Read the model definition and answer for the solid it produces. Units are mm, in the model's axes. A direction names the side the tool comes from. Give positions to 0.01 mm unless a question says otherwise; leave off trailing zeros. Order: outer loops, then holes, each group sorted by start corner. A loop starts at its lowest first (then second) coordinate and runs counter-clockwise, first axis right, second up. Notation, with made-up numbers: (18.5, -13.5) - (36.5, -13.5) arc R23 ccw to (36.5, 2.5) - close; hole circle Ø3 at (-22.75, 13). An arc over 180 degrees is marked (long way). Return JSON: item names as keys, results as strings.
```python
from build123d import *

# Parameters (mm, degrees)
SKETCH1_R           = 1.6
BOSS_EXTRUDE1_DEPTH = 1.65
SKETCH2_W           = 16.5
SKETCH2_H           = 12.1
BOSS_EXTRUDE2_DEPTH = 11


with BuildPart() as part:
    # Sketch1 → Boss-Extrude1 (new body)
    with BuildSketch(Plane(origin=(0, 0, 0), x_dir=(1, 0, 0), z_dir=(0, 1, 0))):
        Polygon((99.1, 0), (99.1, 1), (101.6, 3.5), (101.6, 43.3), (99.1, 45.8), (99.1, 50.8), (96.6, 53.3), (0, 53.3), (0, 0), align=None)
        with Locations((15.524, 50.76)):
            Circle(SKETCH1_R, mode=Mode.SUBTRACT)
        with Locations((14, 2.5)):
            Circle(SKETCH1_R, mode=Mode.SUBTRACT)
        with Locations((96.55, 2.5)):
            Circle(SKETCH1_R, mode=Mode.SUBTRACT)
        with Locations((90.454, 50.76)):
            Circle(SKETCH1_R, mode=Mode.SUBTRACT)
        with Locations((66.1, 35.5)):
            Circle(SKETCH1_R, mode=Mode.SUBTRACT)
        with Locations((66.1, 7.6)):
            Circle(SKETCH1_R, mode=Mode.SUBTRACT)
    extrude(amount=BOSS_EXTRUDE1_DEPTH)

    # Sketch2 → Boss-Extrude2 (add)
    with BuildSketch(Plane(origin=(0, 1.65, 0), x_dir=(1, 0, 0), z_dir=(0, 1, 0))):
        with Locations((2.25, 38.45)):
            Rectangle(SKETCH2_W, SKETCH2_H)
    extrude(amount=BOSS_EXTRUDE2_DEPTH)


solid = part.part
```
Q1. A cutting plane is placed at D-D (y = 7.75). Write down the section's boundary in (x, z).
Values:
{"outline": "(-6, -44.5) - (10.5, -44.5) - (10.5, -32.4) - (-6, -32.4) - close"}
Q2. A cutting plane is placed at C-C (x = 61). Write down the section's boundary in (y, z).
Values:
{"outline": "(0, -53.3) - (1.65, -53.3) - (1.65, 0) - (0, 0) - close"}
Q3. A cutting plane is placed at A-A (z = -35.5). Write down the section's boundary in (x, y).
Values:
{"outline": "(-6, 1.65) - (0, 1.65) - (0, 0) - (64.5, 0) - (64.5, 1.65) - (10.5, 1.65) - (10.5, 12.65) - (-6, 12.65) - close; (67.7, 0) - (101.6, 0) - (101.6, 1.65) - (67.7, 1.65) - close"}
Q4. Determine the mould class of faces 6 (the cylindrical face through (67.626, 0.813, -35.981)), 7 (the cylindrical face through (98.03, 0.81, -1.89)), 8 (the flat face through (2, 12.65, -39)), 9 (the flat face through (-6, 7, -38)) for opening direction X: released by +X, released by -X, zero draft, split by the parting line, or undercut.
Values:
{"face 6": "undercut", "face 7": "undercut", "face 8": "zero draft", "face 9": "released by -X"}
Q5. For faces 1 (the flat face through (10.5, 7, -38)), 2 (the flat face through (-3, 1.65, -39)), 3 (the flat face through (2, 7, -32.4)), 4 (the flat face through (2, 7, -44.5)), 5 (the flat face through (97.9, 0.8, -52)), determine the directions among +Z, -Z, +X, -X, +Y, -Y from which every point of the face is accessible in a straight line to the end or side of a thin tool.
Values:
{"face 1": "+Z, -Z, +X, +Y", "face 2": "+Z, -Z, -X, -Y", "face 3": "+Z, +X, -X, +Y", "face 4": "-Z, +X, -X, +Y", "face 5": "-Z, +X, +Y, -Y"}
Q6. Consider L1, parallel to Z at x = 66.1, y = 0.4; L2, parallel to X at y = 1.05, z = -50.76; L3, parallel to X at y = 0.5, z = -35.5. Determine where each line is inside the solid, lowest interval first.
Values:
{"L1": "z = -53.3 to -37.1, -33.9 to -9.2, -6 to 0", "L2": "x = 0 to 13.92, 17.12 to 88.85, 92.05 to 99.1", "L3": "x = 0 to 64.5, 67.7 to 101.6"}
Q7. A cutting plane is placed at B-B (z = -7.6). Write down the section's boundary in (x, y), and give its area (3 significant figures).
Values:
{"outline": "(0, 0) - (64.5, 0) - (64.5, 1.65) - (0, 1.65) - close; (67.7, 0) - (101.6, 0) - (101.6, 1.65) - (67.7, 1.65) - close", "area": "162 mm²"}
Q8. Given pin 1 (5 mm diameter, centred on x = 14, z = -2.5, fed in from +Y); pin 2 (2 mm diameter, centred on x = 9.5, y = 9, fed in from -Z); pin 3 (1.3 mm diameter, centred on y = 0.5, z = -47, fed in from +X); pin 4 (1.5 mm diameter, centred on x = 46, z = -29, fed in from -Y), each flat-ended and moving along its own axis, determine where each tip first touches the part or whether it passes through.
Values:
{"pin 1": "stops at y = 1.65", "pin 2": "stops at z = -44.5", "pin 3": "stops at x = 99.1", "pin 4": "stops at y = 0"}
